Source: CAD feature listing. Evaluate the final solid. Frame: model axes, mm. Coordinates: 2 decimals unless noted, no trailing zeros. Order: outer loops, then holes, each group sorted by start corner. A loop starts at its lowest first (then second) coordinate and runs counter-clockwise, first axis right, second up.
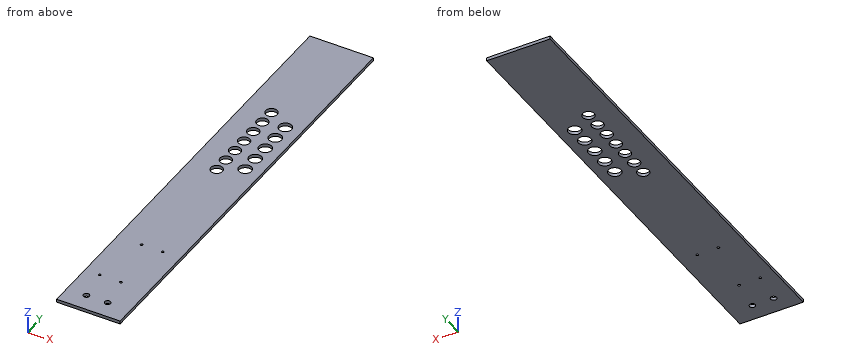
```python
from build123d import *

# Parameters (mm, degrees)
ESQUISSE1_W           = 120
ESQUISSE1_H           = 832
BOSS_EXTRU_1_DEPTH    = 6
M10_CLEARANCE_HOLE1_D = 11
M4_CLEARANCE_HOLE1_D  = 4.5
SKETCH5_R             = 3
CUT_EXTRUDE1_DEPTH    = 10
M20_CLEARANCE_HOLE1_D = 22
M22_CLEARANCE_HOLE1_D = 24
LPATTERN1_COUNT       = 4
LPATTERN1_PITCH       = 30
LPATTERN2_COUNT       = 3
LPATTERN2_PITCH       = 33
LPATTERN3_COUNT       = 3
LPATTERN3_PITCH       = 33
LPATTERN4_COUNT       = 4
LPATTERN4_PITCH       = 30


with BuildPart() as part:
    # Esquisse1 → Boss.-Extru.1 (new body)
    with BuildSketch(Plane.XY):
        Rectangle(ESQUISSE1_W, ESQUISSE1_H)
    extrude(amount=BOSS_EXTRU_1_DEPTH)

    # M10 Clearance Hole1 (through all)
    with Locations(Plane.XY.offset(6)):
        with Locations((17, -382.348938989), (-23, -382.348938989)):
            Hole(M10_CLEARANCE_HOLE1_D / 2)

    # M4 Clearance Hole1 (through all)
    with Locations(Plane.XY.offset(6)):
        with Locations((26, -217), (8, -323), (-32, -323), (-14, -217)):
            Hole(M4_CLEARANCE_HOLE1_D / 2)

    # Sketch5 → Cut-Extrude1 (cut)
    with BuildSketch(Plane.XY.offset(6)):
        with Locations((30, 113)):
            Circle(SKETCH5_R)
        with Locations((-10, 113)):
            Circle(SKETCH5_R)
    extrude(amount=-CUT_EXTRUDE1_DEPTH, mode=Mode.SUBTRACT)

    # M20 Clearance Hole1 (through all)
    with Locations(Plane.XY.offset(6)):
        with Locations((-10, 113)):
            m20_clearance_hole1 = Hole(M20_CLEARANCE_HOLE1_D / 2)

    # M22 Clearance Hole1 (through all)
    with Locations(Plane.XY.offset(6)):
        with Locations((30, 113)):
            m22_clearance_hole1 = Hole(M22_CLEARANCE_HOLE1_D / 2)

    # LPattern1: M20 Clearance Hole1 ×4
    with Locations(*[(0, i * LPATTERN1_PITCH, 0) for i in range(1, LPATTERN1_COUNT)]):
        add(m20_clearance_hole1, mode=Mode.SUBTRACT)

    # LPattern2: M22 Clearance Hole1 ×3
    with Locations(*[(0, i * LPATTERN2_PITCH, 0) for i in range(1, LPATTERN2_COUNT)]):
        add(m22_clearance_hole1, mode=Mode.SUBTRACT)

    # LPattern3: M22 Clearance Hole1 ×3
    with Locations(*[(0, -i * LPATTERN3_PITCH, 0) for i in range(1, LPATTERN3_COUNT)]):
        add(m22_clearance_hole1, mode=Mode.SUBTRACT)

    # LPattern4: M20 Clearance Hole1 ×4
    with Locations(*[(0, -i * LPATTERN4_PITCH, 0) for i in range(1, LPATTERN4_COUNT)]):
        add(m20_clearance_hole1, mode=Mode.SUBTRACT)


solid = part.part
```
Q1. Pin query (flat end, axial travel): P1, Ø19, axis at x = 30, y = 47, coming from the -Z side. Return the tip coordinate at first contact, or that it passes through.
Solutions:
P1: passes through
Q2. Section query B-B on z = 1.45. Give the number of separate pieces and of enclosed holes in the cut face, plus the area to 3 significant figures.
Solutions:
separate pieces: 1
enclosed holes: 18
area: 94,700 mm2
Q3. Material intervals for line 1 along Y through (x, z) = (30, 3.9); line 2 along X through (y, z) = (-217, 3.05); line 3 along Y through (x, z) = (17, 3.3), sorted ascending.
Solutions:
line 1: y = -416 to 35, 59 to 68, 92 to 101, 125 to 134, 158 to 167, 191 to 416
line 2: x = -60 to -16.25, -11.75 to 23.75, 28.25 to 60
line 3: y = -416 to -387.85, -376.85 to 416
Q4. Section query A-A on y = 23. Output: boundary loops of the cut face in (x, z).
Solutions:
outline: (-60, 0) - (-21, 0) - (-21, 6) - (-60, 6) - close; (1, 0) - (60, 0) - (60, 6) - (1, 6) - close
